from build123d import *

# Parameters (mm, degrees)
BOSS_EXTRUDE1_DEPTH = 80
SKETCH2_W           = 30
SKETCH2_H           = 10
BOSS_EXTRUDE2_DEPTH = 5
SKETCH3_W           = 20
SKETCH3_H           = 10
BOSS_EXTRUDE3_DEPTH = 5
BOSS_EXTRUDE4_DEPTH = 5


with BuildPart() as part:
    # Sketch1 → Boss-Extrude1 (new body)
    with BuildSketch(Plane.XY):
        with BuildLine():
            Line((-10, 0), (-10, 10))
            Line((-10, 10), (-12, 10))
            Line((-12, 10), (-12, 0))
            ThreePointArc((-12, 0), (0, -12), (12, 0))
            Line((12, 0), (12, 10))
            Line((12, 10), (10, 10))
            Line((10, 10), (10, 0))
            ThreePointArc((10, 0), (0, -10), (-10, 0))
        make_face()
    extrude(amount=BOSS_EXTRUDE1_DEPTH)

    # Sketch2 → Boss-Extrude2 (add)
    with BuildSketch(Plane(origin=(0, 0, 0), x_dir=(-1, 0, 0), z_dir=(0, 0, -1))):
        with Locations((25, 5)):
            Rectangle(SKETCH2_W, SKETCH2_H)
    extrude(amount=-BOSS_EXTRUDE2_DEPTH)

    # Sketch3 → Boss-Extrude3 (add)
    with BuildSketch(Plane(origin=(0, 0, 0), x_dir=(-1, 0, 0), z_dir=(0, 0, -1))):
        with Locations((30, 5)):
            Rectangle(SKETCH3_W, SKETCH3_H)
    extrude(amount=BOSS_EXTRUDE3_DEPTH)

    # Sketch4 → Boss-Extrude4 (add)
    with BuildSketch(Plane.XZ):
        Polygon((-12, 0), (-12, 5), (-40, 5), (-40, -5), (-20, -5), (-20, 0), align=None)
    extrude(amount=BOSS_EXTRUDE4_DEPTH)


solid = part.part
For this review, take the finished solid that the model builds, in its own axes (mm). A direction names the side the tool comes from. Give positions to 0.01 mm unless a question says otherwise; leave off trailing zeros. Write each loop counter-clockwise with the first axis right and the second up, starting at its lowest first coordinate (ties: lowest second). Pieces come first, ordered by that corner, then holes. Notation, with made-up numbers: (-7, 16.25) -> (17, 16.25) arc R17 cw to (17, 42.25) -> close; hole circle Ø7 at (-12.5, 73). An arc over 180 degrees is marked (long way). Use CSV: the item, a comma, the result in double quotes.
Q1. Take a section at C-C, the plane x = -26.5. Write out the cut boundary in (y, z), then the cut area to 3 significant figures.
Conclusion:
outline,"(-5, -5) -> (10, -5) -> (10, 5) -> (-5, 5) -> close"
area,"150 mm2"
Q2. Take a section at B-B, the plane z = 3. Write out the cut boundary in (x, y).
Conclusion:
outline,"(-40, -5) -> (-12, -5) -> (-12, 0) arc R12 ccw to (12, 0) -> (12, 10) -> (10, 10) -> (10, 0) arc R10 cw to (-10, 0) -> (-10, 10) -> (-40, 10) -> close"
Q3. For P1, Ø1.5, axis at y = -1.5, z = 2.5, coming from the +X side; P2, Ø1.5, axis at y = -1, z = -3.5, coming from the +X side; P3, Ø3, axis at x = -27, z = 0, coming from the -Y side, all flat-tipped, find the tip position at first contact; note any pin that passes through.
Conclusion:
P1,"x = 11.98"
P2,"x = -20"
P3,"y = -5"
Q4. To check wall thickness, follow probe 1 along X at (y, z) = (7.5, 46); probe 2 along X at (y, z) = (-3.75, 70.5); probe 3 along Z at (x, y) = (-34, 6.5). State the ranges of each line that lie inside material, in increasing order. Write a range as [from, to].
Conclusion:
probe 1,"[-12, -10], [10, 12]"
probe 2,"[-11.4, -9.27], [9.27, 11.4]"
probe 3,"[-5, 5]"
Q5. Tool access review of faces 1 (the face through (-20, 3, -3)), 2 (the face through (-29, -5, 0)), 3 (the face through (-10, 5, 39)), 4 (the face through (-12, 5, 42)), 5 (the face through (-30, 3, -5)): name each direction out of +Z, -Z, +X, -X, +Y, -Y from which nothing blocks a thin tool from reaching the whole face with its end or side.
Conclusion:
face 1,"-Z, +X, +Y, -Y"
face 2,"+Z, -Z, -X, -Y"
face 3,"+Z, -Z, +Y"
face 4,"+Z, -X, +Y, -Y"
face 5,"-Z, +X, -X, +Y, -Y"
Q6. Take a section at A-A, the plane y = 2.5. Write out the cut boundary in (x, z), then the cut area to 3 significant figures.
Conclusion:
outline,"(-40, -5) -> (-20, -5) -> (-20, 0) -> (-10, 0) -> (-10, 80) -> (-12, 80) -> (-12, 5) -> (-40, 5) -> close; (10, 0) -> (12, 0) -> (12, 80) -> (10, 80) -> close"
area,"560 mm2"
Q7. Take a section at D-D, the plane z = 41.5. Write out the cut boundary in (x, y), then the cut area to 3 significant figures.
Conclusion:
outline,"(-12, 0) arc R12 ccw to (12, 0) -> (12, 10) -> (10, 10) -> (10, 0) arc R10 cw to (-10, 0) -> (-10, 10) -> (-12, 10) -> close"
area,"109 mm2"
